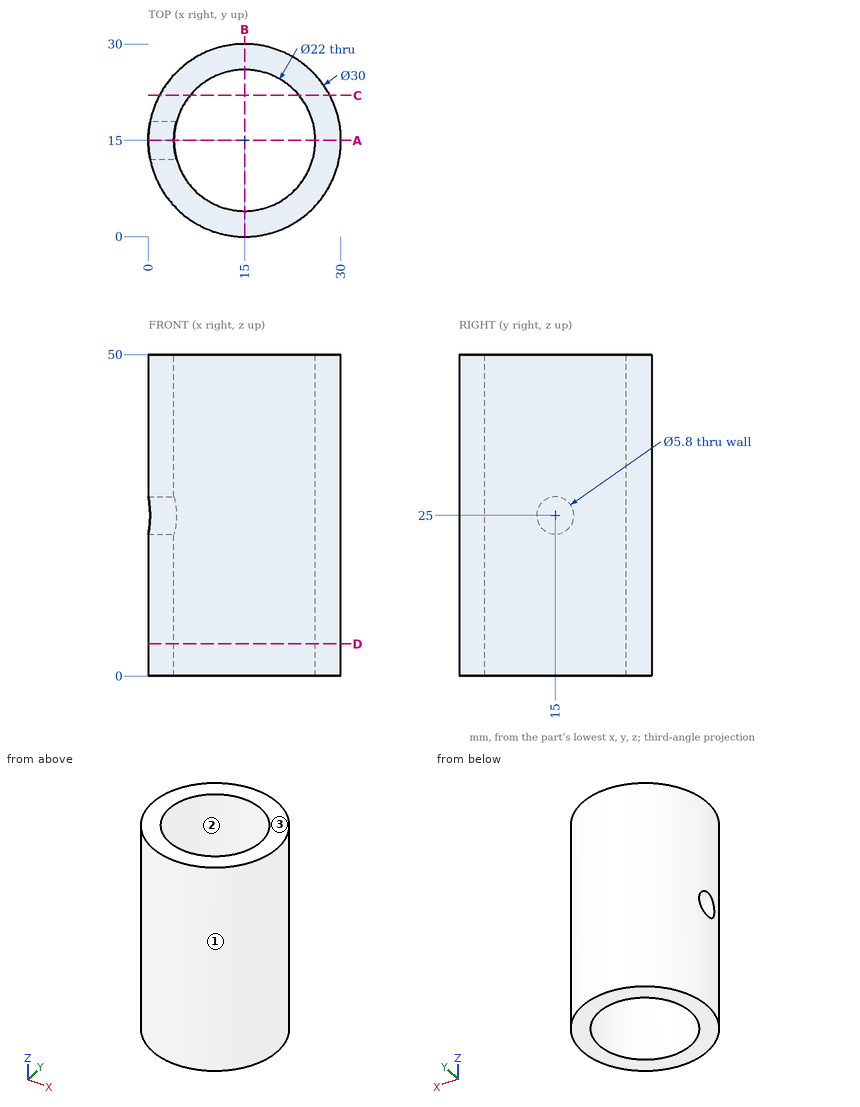
Source: three-view drawing plus pictorial views. Frame: mm from the lowest corner of the part. Round coordinates to 2 decimals unless told otherwise and drop trailing zeros. Order: outer loops, then holes, each group sorted by start corner. A loop starts at its lowest first (then second) coordinate and runs counter-clockwise, first axis right, second up. Notation, with made-up numbers: (-38.5, 20) - (-10.5, 20) arc R36 cw to (-10.5, 57) - close; hole circle Ø7 at (33, -35). An arc over 180 degrees is marked (long way). Answer in a Markdown table with one row per item.
Item 1: Mould query, pull axis X, two halves, no side actions, for the marked faces 1, 2 and 3. Classes: released by +X, released by -X, zero draft, split by the parting line, or undercut.
Model answer:
| item | result |
|---|---|
| face 1 | split by the parting line |
| face 2 | undercut |
| face 3 | zero draft |
Item 2: Section query D-D (z = 5). Return the cut outline in (x, y), then the cut area to 3 significant figures.
Model answer:
| item | result |
|---|---|
| outline | circle Ø30 at (15, 15); hole circle Ø22 at (15, 15) |
| area | 327 mm² |
Item 3: Line query: line 1 (Y direction, x = 15, z = 14); line 2 (X direction, y = 18.5, z = 8.5); line 3 (Y direction, x = 20, z = 43). Output: solid intervals per line, ascending.
Model answer:
| item | result |
|---|---|
| line 1 | y = 0 to 4, 26 to 30 |
| line 2 | x = 0.41 to 4.57, 25.43 to 29.59 |
| line 3 | y = 0.86 to 5.2, 24.8 to 29.14 |
Item 4: Section query C-C (y = 22). Return the cut outline in (x, z).
Model answer:
| item | result |
|---|---|
| outline | (1.73, 0) - (6.51, 0) - (6.51, 50) - (1.73, 50) - close; (23.49, 0) - (28.27, 0) - (28.27, 50) - (23.49, 50) - close |
Item 5: Pin query (flat end, axial travel): pin 1 (1.5 mm diameter, centred on x = 3.5, z = 7, fed in from -Y); pin 2 (5 mm diameter, centred on y = 10.5, z = 21, fed in from +X); pin 3 (8 mm diameter, centred on x = 9, z = 12.5, fed in from +Y); pin 4 (5 mm diameter, centred on x = 16, z = 42, fed in from -Y). Return the tip coordinate at first contact, or that it passes through.
Model answer:
| item | result |
|---|---|
| pin 1 | stops at y = 4.54 |
| pin 2 | stops at x = 29.87 |
| pin 3 | stops at y = 29.87 |
| pin 4 | stops at y = 0 |
Item 6: Section query B-B (x = 15). Return the cut outline in (y, z), then the cut area to 3 significant figures.
Model answer:
| item | result |
|---|---|
| outline | (0, 0) - (4, 0) - (4, 50) - (0, 50) - close; (26, 0) - (30, 0) - (30, 50) - (26, 50) - close |
| area | 400 mm² |
Item 7: Section query A-A (y = 15). Return the cut outline in (x, z), then the cut area to 3 significant figures.
Model answer:
| item | result |
|---|---|
| outline | (0, 0) - (4, 0) - (4, 22.1) - (0, 22.1) - close; (0, 27.9) - (4, 27.9) - (4, 50) - (0, 50) - close; (26, 0) - (30, 0) - (30, 50) - (26, 50) - close |
| area | 377 mm² |
